Geometry check sheet. Reference: the model listing, model coordinates, mm. Face numbers are marked on the shaded views. A direction names the side the tool comes from. Round coordinates to 2 decimals unless told otherwise and drop trailing zeros. Order: outer loops, then holes, each group sorted by start corner. A loop starts at its lowest first (then second) coordinate and runs counter-clockwise, first axis right, second up.
(1) Sectioned sample at B-B (x = 1). Record the boundary of the cut face in (y, z), plus the area to 3 significant figures.
(2) Material ranges on line 1 along Y through (x, z) = (2, 9); line 2 along X through (y, z) = (-34.5, 22); line 3 along X through (y, z) = (13.5, 5.5), recorded low to high.
(3) Release check for a two-part mould opening along Y. For the marked faces 1, 2, 3 and 4 record: +Y half, -Y half, draft (parallel to the pull), parting line (faces both ways), or undercut.
(4) Go/stop test with flat-tipped pins: pin 1 (1 mm diameter, centred on x = 3, z = 15.5, fed in from +Y); pin 2 (3 mm diameter, centred on x = -6.09, z = 22.52, fed in from +Y); pin 3 (4 mm diameter, centred on x = 28, y = 1.5, fed in from +Z); pin 4 (5 mm diameter, centred on y = -23.5, z = 10.5, fed in from -X). Record where each tip stops, or that it passes through.
(5) Sectioned sample at A-A (z = 18). Record the boundary of the cut face in (x, y).
(6) Sectioned sample at D-D (x = 10.5). Record the boundary of the cut face in (y, z), plus the area to 3 significant figures.
(7) Sectioned sample at C-C (y = 18). Record the boundary of the cut face in (x, z).
(8) Set-up check for the marked faces 5, 6, 7, 8 and 9: record each of +Z, -Z, +X, -X, +Y, -Y from which the full face is reachable in a straight line by a thin tool's end or side.
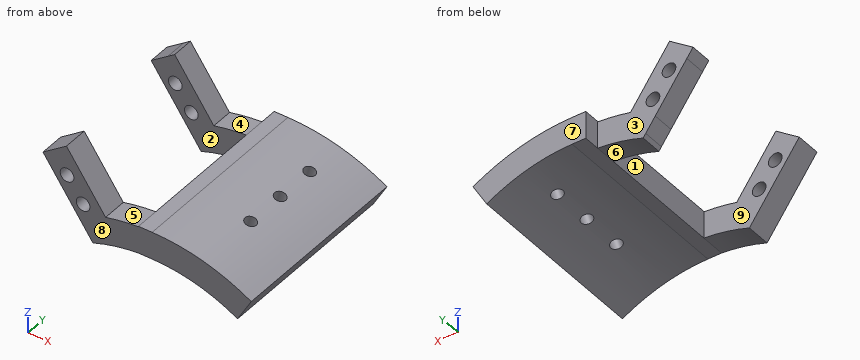
from build123d import *

# Parameters (mm, degrees)
BOSS_EXTRUDE2_DEPTH = 20
FILLET1_RADIUS      = 10
FILLET1_LENGTH      = 5
FILLET2_RADIUS      = 10
FILLET2_LENGTH      = 5
SKETCH5_R           = 1
SKETCH5_R_2         = 5.5
CUT_EXTRUDE5_DEPTH  = 69.007352544
CUT_EXTRUDE7_DEPTH  = 25
FILLET5_R           = 10
BOSS_EXTRUDE5_DEPTH = 60
SKETCH13_R          = 2.1
CUT_EXTRUDE8_DEPTH  = 60
CUT_EXTRUDE9_DEPTH  = 60
CUT_EXTRUDE10_DEPTH = 60
SKETCH17_R          = 2.5
BOSS_EXTRUDE6_DEPTH = 8
SKETCH18_R          = 2.5
BOSS_EXTRUDE7_DEPTH = 9


with BuildPart() as part:
    # Sketch1 → Boss-Extrude2 (new body)
    with BuildSketch(Plane.XY):
        Polygon((-25, 30), (25, 30), (25, -30), (-25, -30), (-25, -25), (-20, -25), (20, -25), (20, 25), (-20, 25), (-25, 25), align=None)
    extrude(amount=BOSS_EXTRUDE2_DEPTH)

    # Fillet1: full round fillet: the end face becomes a half cylinder, R = half its width
    fillet1_face = Plane((-25, 27.5, 10), x_dir=(0, -1, 0), z_dir=(-1, 0, 0))  # on the end face: x along it, z out of the body
    fillet1_slab = fillet1_face.offset(-FILLET1_RADIUS / 2) * Box(FILLET1_LENGTH, 2 * FILLET1_RADIUS, FILLET1_RADIUS, mode=Mode.PRIVATE)  # the body's end, R deep
    fillet1_round = Plane((-15, 27.5, 10), x_dir=(-1, 0, 0), z_dir=(0, -1, 0)) * Cylinder(FILLET1_RADIUS, FILLET1_LENGTH, mode=Mode.PRIVATE)  # its axis R under the face
    add(fillet1_slab - fillet1_round, mode=Mode.SUBTRACT)

    # Fillet2: full round fillet: the end face becomes a half cylinder, R = half its width
    fillet2_face = Plane((-25, -27.5, 10), x_dir=(0, -1, 0), z_dir=(-1, 0, 0))  # on the end face: x along it, z out of the body
    fillet2_slab = fillet2_face.offset(-FILLET2_RADIUS / 2) * Box(FILLET2_LENGTH, 2 * FILLET2_RADIUS, FILLET2_RADIUS, mode=Mode.PRIVATE)  # the body's end, R deep
    fillet2_round = Plane((-15, -27.5, 10), x_dir=(-1, 0, 0), z_dir=(0, -1, 0)) * Cylinder(FILLET2_RADIUS, FILLET2_LENGTH, mode=Mode.PRIVATE)  # its axis R under the face
    add(fillet2_slab - fillet2_round, mode=Mode.SUBTRACT)

    # Sketch5 → Cut-Extrude5 (cut, through all)
    with BuildSketch(Plane(origin=(0, 30, 0), x_dir=(1, 0, 0), z_dir=(0, 1, 0))):
        with Locations(Location((-15, -3, 0), (0, 0, 180))):
            Circle(SKETCH5_R)
        with Locations(Location((-22, -10, 0), (0, 0, 180))):
            Circle(SKETCH5_R)
        with Locations(Location((-15, -17, 0), (0, 0, 180))):
            Circle(SKETCH5_R)
        with Locations(Location((-8, -10, 0), (0, 0, 180))):
            Circle(SKETCH5_R)
        with Locations(Location((-15, -10, 0), (0, 0, 180))):
            Circle(SKETCH5_R_2)
    extrude(amount=-CUT_EXTRUDE5_DEPTH, mode=Mode.SUBTRACT)

    # Sketch10 → Cut-Extrude7 (cut)
    with BuildSketch(Plane(origin=(25, 0, 0), x_dir=(0, 0, -1), z_dir=(1, 0, 0))):
        Polygon((-15, 28.180148829), (-15, -28.180148829), (-15, -30), (-20, -30), (-20, 30), (-15, 30), align=None)
        Polygon((-5, 28.180148829), (-5, -28.180148829), (-5, -30), (0, -30), (0, 30), (-5, 30), align=None)
    extrude(amount=-CUT_EXTRUDE7_DEPTH, mode=Mode.SUBTRACT)

    # Fillet5
    # the kernel refuses this fillet: 10 mm, written as the material it adds along each edge
    with BuildSketch(Plane(origin=(0, 25, 15), x_dir=(1, 0, 0), z_dir=(0, 1, 0)), Plane(origin=(0, -30, 15), x_dir=(1, 0, 0), z_dir=(0, 1, 0)), Plane(origin=(0, -25, 5), x_dir=(1, 0, 0), z_dir=(0, -1, 0))) as fillet5_piece_1:
        with BuildLine():
            CenterArc((8.660254038, -10), FILLET5_R, 90, 60)
            Line((0, -5), (-0.173205081, -4.9))
            ThreePointArc((-0.173205081, -4.9), (-0.2, -2.5), (-0.2, 0))
            Line((-0.2, 0), (0, 0.2))
            Line((0, 0.2), (8.660254038, 0.2))
            Line((8.660254038, 0.2), (8.660254038, 0))
        make_face()
    extrude(amount=5)
    with BuildSketch(Plane(origin=(0, 30, 5), x_dir=(0, 0, -1), z_dir=(0, -1, 0))) as fillet5_piece_2:
        with BuildLine():
            CenterArc((10, 8.660254038), FILLET5_R, 180, 60)
            Line((0, 8.660254038), (-0.2, 8.660254038))
            Line((-0.2, 8.660254038), (-0.2, 0))
            Line((-0.2, 0), (0, -0.2))
            ThreePointArc((0, -0.2), (2.5, -0.2), (4.9, -0.173205081))
            Line((4.9, -0.173205081), (5, 0))
        make_face()
    extrude(amount=5)

    # Sketch12 → Boss-Extrude5 (add)
    with BuildSketch(Plane.XZ.offset(30)):
        with BuildLine():
            Line((56.226298398, -3.359735054), (61.222506141, 5.302707337))
            ThreePointArc((61.222506141, 5.302707337), (43.74904955, 12.533728595), (25, 15))
            Line((25, 15), (25, 5))
            ThreePointArc((25, 5), (41.16297375, 2.873903962), (56.226298398, -3.359735054))
        make_face()
    extrude(amount=-BOSS_EXTRUDE5_DEPTH)

    # Sketch13 → Cut-Extrude8 (cut)
    with BuildSketch(Plane(origin=(2.920998947, 0, 10.910870277), x_dir=(-0.9659824633840055, 0, 0.2586075800021504), z_dir=(-0.2586075800021504, 0, -0.9659824633840055))):
        with Locations((-39.019497435, 15)):
            Circle(SKETCH13_R)
        with Locations((-39.019497435, 0)):
            Circle(SKETCH13_R)
        with Locations((-39.019497435, -15)):
            Circle(SKETCH13_R)
    extrude(amount=-CUT_EXTRUDE8_DEPTH, mode=Mode.SUBTRACT)

    # Sketch15 → Cut-Extrude9 (cut)
    with BuildSketch(Plane(origin=(0, 30, 0), x_dir=(1, 0, 0), z_dir=(0, 1, 0))):
        with BuildLine():
            Line((8.660254038, -5), (8.660254038, -15))
            ThreePointArc((8.660254038, -15), (-39.182795974, -10), (8.660254038, -5))
        make_face()
    extrude(amount=-CUT_EXTRUDE9_DEPTH, mode=Mode.SUBTRACT)

    # Sketch16 → Cut-Extrude10 (cut)
    with BuildSketch(Plane(origin=(0, 30, 0), x_dir=(1, 0, 0), z_dir=(0, 1, 0))):
        Polygon((-6.307906019, -33.220384693), (8.660254038, -15), (20.000254038, -15), (20.000254038, -5), (8.660254038, -5), (3.496355525, -1.350438774), (-14.790578774, -27.225295226), align=None)
    extrude(amount=-CUT_EXTRUDE10_DEPTH, mode=Mode.SUBTRACT)

    # Sketch17 → Boss-Extrude6 (add)
    # profile 1 of 2: a face of its own
    with BuildSketch(Plane(origin=(0, 16, 0), x_dir=(1, 0, 0), z_dir=(0, 1, 0))):
        Polygon((2.432023453, -2.661202229), (-1.062108246, -7.605177784), (-12.605177784, -23.937891754), (-14.882580853, -27.160273185), (-8.757813114, -31.488924262), (-6.307906019, -33.220384693), (7.998117102, -12.978265997), (11.006698288, -8.721313737), align=None)
        with Locations(Location((-6.090722034, -22.517234763, 0), (0, 0, 180))):
            Circle(SKETCH17_R, mode=Mode.SUBTRACT)
        with Locations(Location((-0.226842709, -14.220216066, 0), (0, 0, 180))):
            Circle(SKETCH17_R, mode=Mode.SUBTRACT)
    # profile 2 of 2: a face of its own
    with BuildSketch(Plane(origin=(0, 16, 0), x_dir=(1, 0, 0), z_dir=(0, 1, 0))):
        with BuildLine():
            Line((3.360713643, -1.347164296), (2.432023453, -2.661202229))
            Line((2.432023453, -2.661202229), (11.006698288, -8.721313737))
            Line((11.006698288, -8.721313737), (7.998117102, -12.978265997))
            ThreePointArc((7.998117102, -12.978265997), (13.960401245, -14.154569005), (20.000254038, -14.827398269))
            Line((20.000254038, -14.827398269), (20.000254038, -5))
            ThreePointArc((20.000254038, -5), (11.555844657, -3.741343444), (3.360713643, -1.347164296))
        make_face()
    extrude(amount=BOSS_EXTRUDE6_DEPTH)

    # Sketch18 → Boss-Extrude7 (add)
    with BuildSketch(Plane(origin=(0, -39, 0), x_dir=(1, 0, 0), z_dir=(0, 1, 0))):
        with BuildLine():
            Line((3.360713643, -1.347164296), (-14.882580853, -27.160273185))
            Line((-14.882580853, -27.160273185), (-6.307906019, -33.220384693))
            Line((-6.307906019, -33.220384693), (7.998117102, -12.978265997))
            ThreePointArc((7.998117102, -12.978265997), (13.960401245, -14.154569005), (20.000254038, -14.827398269))
            Line((20.000254038, -14.827398269), (20.000254038, -15))
            Line((20.000254038, -15), (25, -15))
            ThreePointArc((25, -15), (43.74904955, -12.533728595), (61.222506141, -5.302707337))
            Line((61.222506141, -5.302707337), (56.226298398, 3.359735054))
            ThreePointArc((56.226298398, 3.359735054), (41.16297375, -2.873903962), (25, -5))
            Line((25, -5), (20.000254038, -5))
            ThreePointArc((20.000254038, -5), (11.555844657, -3.741343444), (3.360713643, -1.347164296))
        make_face()
        with Locations(Location((-6.090722034, -22.517234763, 0), (0, 0, 180))):
            Circle(SKETCH18_R, mode=Mode.SUBTRACT)
        with Locations(Location((-0.226842709, -14.220216066, 0), (0, 0, 180))):
            Circle(SKETCH18_R, mode=Mode.SUBTRACT)
    extrude(amount=BOSS_EXTRUDE7_DEPTH)


solid = part.part
Answer below:
1. outline: (-39, 4.69) - (-30, 4.69) - (-30, 12.04) - (-39, 12.04) - close; (-39, 16.4) - (-30, 16.4) - (-30, 22.88) - (-39, 22.88) - close; (16, 4.69) - (24, 4.69) - (24, 12.04) - (16, 12.04) - close; (16, 16.4) - (24, 16.4) - (24, 22.88) - (16, 22.88) - close
1. area: 235 mm2
2. line 1: y = -39 to -30, 16 to 24
2. line 2: x = -11.24 to -8.54, -3.64 to 1.62
2. line 3: x = 20 to 40.34, 43.39 to 60.88
3. face 1: undercut
3. face 2: undercut
3. face 3: +Y half
3. face 4: draft
4. pin 1: stops at y = 24
4. pin 2: passes through
4. pin 3: stops at z = 14.99
4. pin 4: stops at x = 20
5. outline: (-8.41, -39) - (4.45, -39) - (4.45, -30) - (-8.41, -30) - close; (-8.41, 16) - (4.45, 16) - (4.45, 24) - (-8.41, 24) - close
6. outline: (-39, 3.5) - (-30, 3.5) - (-30, 13.54) - (-39, 13.54) - close; (16, 3.5) - (24, 3.5) - (24, 13.54) - (16, 13.54) - close
6. area: 171 mm2
7. outline: (-14.88, 27.16) - (3.36, 1.35) arc R62.7 cw to (20, 5) - (25, 5) arc R62.5 cw to (56.23, -3.36) - (61.22, 5.3) arc R72.5 ccw to (25, 15) - (20, 15) - (20, 14.83) arc R72.5 ccw to (8, 12.98) - (-6.31, 33.22) - close; hole circle Ø5 at (-6.09, 22.52); hole circle Ø5 at (-0.23, 14.22)
8. face 5: +Z, +Y, -Y
8. face 6: -Z, +Y, -Y
8. face 7: +Z, -Z, +X, -X, +Y
8. face 8: +Z, -Z, +X, -X, -Y
8. face 9: +Z, -Z, -X
